from build123d import *

# Parameters (mm, degrees)
SKETCH1_R           = 19.05
SKETCH1_R_2         = 11.1125
BOSS_EXTRUDE1_DEPTH = 76.2
SKETCH2_R           = 16.66875
SKETCH2_R_2         = 11.1125
BOSS_EXTRUDE2_DEPTH = 31.75
CUT_EXTRUDE1_DEPTH  = 77.2


with BuildPart() as part:
    # Sketch1 → Boss-Extrude1 (new body)
    with BuildSketch(Plane(origin=(0, 0, 0), x_dir=(1, 0, 0), z_dir=(0, 1, 0))):
        Circle(SKETCH1_R)
        Circle(SKETCH1_R_2, mode=Mode.SUBTRACT)
    extrude(amount=BOSS_EXTRUDE1_DEPTH)

    # Sketch2 → Boss-Extrude2 (add)
    with BuildSketch(Plane(origin=(0, 76.2, 0), x_dir=(1, 0, 0), z_dir=(0, 1, 0))):
        Circle(SKETCH2_R)
        Circle(SKETCH2_R_2, mode=Mode.SUBTRACT)
    extrude(amount=BOSS_EXTRUDE2_DEPTH)

    # Sketch3 → Cut-Revolve1 (revolve, cut)
    with BuildSketch(Plane(origin=(0, 0, 0), x_dir=(0, 0, -1), z_dir=(1, 0, 0))):
        Polygon((16.66875, 107.95), (16.66875, 100.57660721), (11.1125, 107.95), align=None)
    revolve(axis=Axis((0, 107.95, 0), (0, 1, 0)), mode=Mode.SUBTRACT)

    # Sketch4 → Cut-Extrude1 (cut, through all)
    with BuildSketch(Plane(origin=(0, 76.2, 0), x_dir=(1, 0, 0), z_dir=(0, 1, 0))):
        with BuildLine():
            Line((24.271104702, -16.66875), (-24.271104702, -16.66875))
            ThreePointArc((-24.271104702, -16.66875), (0, -29.443738723), (24.271104702, -16.66875))
        make_face()
    extrude(amount=-CUT_EXTRUDE1_DEPTH, mode=Mode.SUBTRACT)

    # Sketch8 → Cut-Revolve4 (revolve, cut)
    with BuildSketch(Plane.XY):
        with BuildLine():
            Line((0, 0), (-6.35, 0))
            add(Edge.make_bspline(
                [(-19.05, 3.175), (-19.05, 0), (-6.35, 0)],
                knots=[3.141592654, 3.141592654, 3.141592654, 4.71238898, 4.71238898, 4.71238898], degree=2, weights=[1, 0.707106781, 1]))
            Line((-19.05, 3.175), (-19.05, -4.469484217))
            Line((-19.05, -4.469484217), (0, -4.469484217))
            Line((0, -4.469484217), (0, 0))
        make_face()
    revolve(axis=Axis((0, 0, 0), (0, 1, 0)), mode=Mode.SUBTRACT)


solid = part.part
Can you work these out from the model? Positions are in its coordinate system, mm. Coordinates: 2 decimals unless noted, no trailing zeros. Loops run counter-clockwise (first coordinate to the right, second up) from the corner with the lowest first, then second, coordinate; pieces in that order, holes last. Notation, with made-up numbers: M -27.5,83 L -19.5,83 A20 ccw -19.5,109 Z; hole C 49,64.5 d9. An arc over 180 degrees is marked long. Return JSON: item names as keys, results as strings. Group by question number.
Item 1: Imagine slicing it at B-B (y = 99). Please give me the cut outline in (x, z) (1 decimal).
Item 2: I'm going to push flat-ended pins straight in: pin 1 Ø2 at (x, y) = (9.5, 91) entering from +Z; pin 2 Ø1 at (y, z) = (67, -13.5) entering from +X; pin 3 Ø1.5 at (x, z) = (4, -15.5) entering from -Y. Where does each tip first touch, or does it pass through?
Item 3: Thinking about a two-plate mould opening in Z: for faces 1 (the cylindrical face through (10.6, 53.34, -3.34)), 2 (the flat face through (0, 39, 16.669)), 3 (the cylindrical face through (0.703, 39.176, -19.037)), 4 (the flat face through (6, 76.2, -16)), which applies, released by +Z, released by -Z, zero draft, split by the parting line, or undercut?
Item 4: If I drill on L1, parallel to X at y = 39, z = 0; L2, parallel to Z at x = 0, y = 24; L3, parallel to X at y = 82, z = 0, over which ranges is the centre line in solid material (lowest first)? Write a range as from..to.
Verdict:
{
 "1": {"outline": "C 0,0 d33.3; hole C 0,0 d22.2"},
 "2": {"pin 1": "stops at z = 14.34", "pin 2": "stops at x = 13.92", "pin 3": "stops at y = 0.91"},
 "3": {"face 1": "undercut", "face 2": "released by +Z", "face 3": "split by the parting line", "face 4": "zero draft"},
 "4": {"L1": "x = -19.05..-11.11, 11.11..19.05", "L2": "z = -19.05..-11.11, 11.11..16.67", "L3": "x = -16.67..-11.11, 11.11..16.67"}
}
